Answer from the drawing. Dimensions are ordinates in mm from the lowest x, y and z of the part. A direction names the side the tool comes from. Coordinates: 2 decimals unless noted, no trailing zeros. Write each loop counter-clockwise with the first axis right and the second up, starting at its lowest first coordinate (ties: lowest second). Pieces come first, ordered by that corner, then holes. Notation, with made-up numbers: (-35, 47.25) - (-17, 47.25) arc R27 ccw to (-17, 79.25) - close; hole circle Ø7 at (25.5, 18). An arc over 180 degrees is marked (long way). Answer as a JSON object with one key per item and string values. Group by question number.
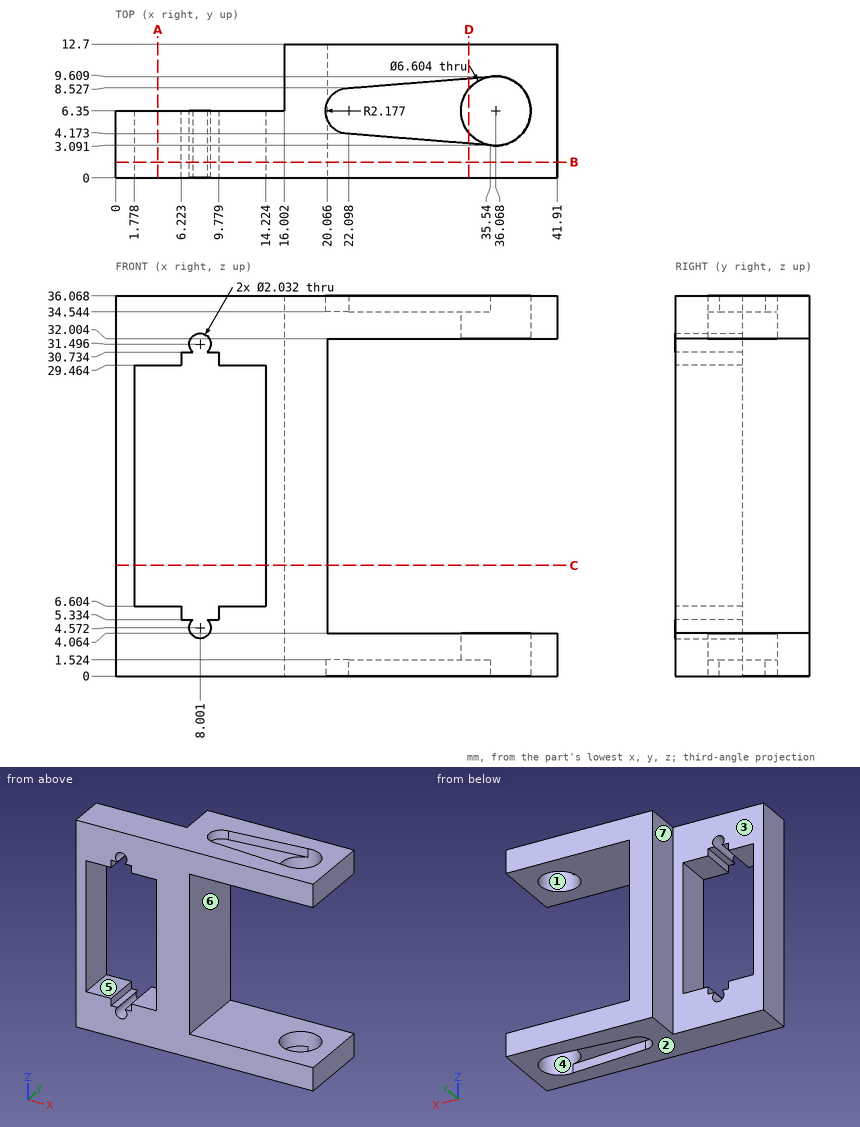
Q1. Section B-B on y = 1.5 is taken. Determine the outline of the cut face in (x, z).
Q2. Section D-D on x = 33.5 is taken. Determine the outline of the cut face in (y, z) (1 decimal).
Q3. A tool of negligible diameter and unlimited length cuts with its end or side. For the marked faces 5, 6 and 7, from which of +Z, -Z, +X, -X, +Y, -Y can it reach the whole face along a straight path? Write none if from no direction.
Q4. Section A-A on x = 4 is taken. Determine the outline of the cut face in (y, z).
Q5. Section C-C on z = 10.5 is taken. Determine the outline of the cut face in (x, y).
Q6. Flat-ended cylindrical pins translate along their axes: pin 1 Ø1 at (y, z) = (4.5, 30) entering from +X; pin 2 Ø5 at (x, y) = (26, 5.5) entering from +Z; pin 3 Ø6 at (x, z) = (4.5, 30) entering from +Y; pin 4 Ø3 at (y, z) = (11, 21.5) entering from -X. Find the tip coordinate at first contact, or state that the pin passes through.
Q7. For a pull along Y with two mould halves and no side action, classify the marked faces 1, 2, 3 and 4 as +Y half, -Y half, draft (parallel to the pull), parting line (faces both ways), or undercut.
Q8. Consider L1, parallel to Z at x = 3, y = 3.75; L2, parallel to Z at x = 37.5, y = 12; L3, parallel to X at y = 2.25, z = 14.5. Determine where each line is inside the solid, lowest interval first. Write a range as from..to.
Numbers:
{
 "1": {"outline": "(0, 0) - (41.91, 0) - (41.91, 4.06) - (20.07, 4.06) - (20.07, 32) - (41.91, 32) - (41.91, 36.07) - (0, 36.07) - close; hole (1.78, 6.6) - (6.22, 6.6) - (6.22, 5.33) - (7.33, 5.33) arc R1.02 ccw (long way) to (8.67, 5.33) - (9.78, 5.33) - (9.78, 6.6) - (14.22, 6.6) - (14.22, 29.46) - (9.78, 29.46) - (9.78, 30.73) - (8.67, 30.73) arc R1.02 ccw (long way) to (7.33, 30.73) - (6.22, 30.73) - (6.22, 29.46) - (1.78, 29.46) - close"},
 "2": {"outline": "(0, 0) - (3.3, 0) - (3.3, 1.5) - (4.3, 1.5) - (4.3, 4.1) - (0, 4.1) - close; (0, 32) - (4.3, 32) - (4.3, 34.5) - (3.3, 34.5) - (3.3, 36.1) - (0, 36.1) - close; (8.4, 1.5) - (9.4, 1.5) - (9.4, 0) - (12.7, 0) - (12.7, 4.1) - (8.4, 4.1) - close; (8.4, 32) - (12.7, 32) - (12.7, 36.1) - (9.4, 36.1) - (9.4, 34.5) - (8.4, 34.5) - close"},
 "3": {"face 5": "+Y, -Y", "face 6": "+X, +Y, -Y", "face 7": "+Z, -Z, -X, +Y"},
 "4": {"outline": "(0, 0) - (6.35, 0) - (6.35, 6.6) - (0, 6.6) - close; (0, 29.46) - (6.35, 29.46) - (6.35, 36.07) - (0, 36.07) - close"},
 "5": {"outline": "(0, 0) - (1.78, 0) - (1.78, 6.35) - (0, 6.35) - close; (14.22, 0) - (20.07, 0) - (20.07, 12.7) - (16, 12.7) - (16, 6.35) - (14.22, 6.35) - close"},
 "6": {"pin 1": "stops at x = 20.07", "pin 2": "stops at z = 36.07", "pin 3": "stops at y = 6.35", "pin 4": "stops at x = 16"},
 "7": {"face 1": "undercut", "face 2": "draft", "face 3": "+Y half", "face 4": "undercut"},
 "8": {"L1": "z = 0..6.6, 29.46..36.07", "L2": "z = 0..4.06, 32..36.07", "L3": "x = 0..1.78, 14.22..20.07"}
}
